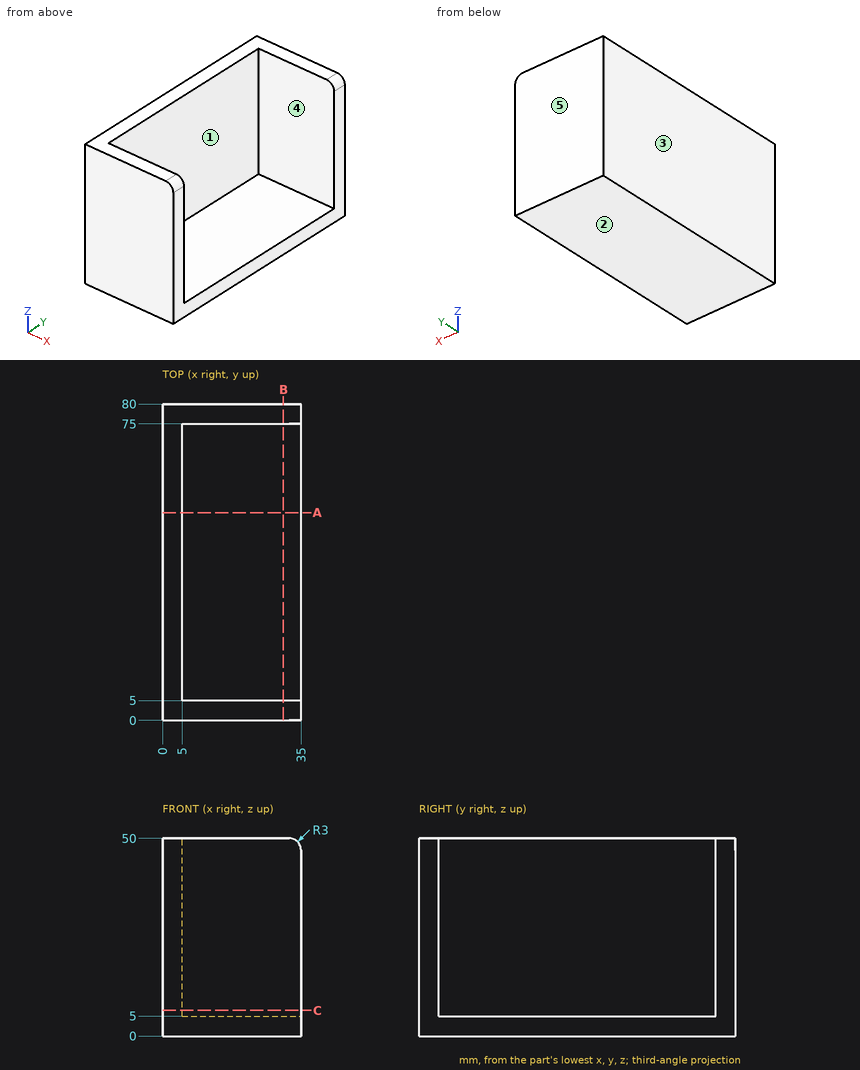
Here's the drawing with two shaded views (mm, measured from the low corner). I have some questions. A direction names the side the tool comes from. Round coordinates to 2 decimals unless told otherwise and drop trailing zeros. Loops run counter-clockwise (first coordinate to the right, second up) from the corner with the lowest first, then second, coordinate; pieces in that order, holes last.
1. Suppose I cut it at B-B, the plane x = 30.5. Please give me the cut outline in (y, z).
Answers:
outline: (0, 0) - (80, 0) - (80, 50) - (75, 50) - (75, 5) - (5, 5) - (5, 50) - (0, 50) - close
2. Suppose I cut it at C-C, the plane z = 6.5. Please give me the cut outline in (x, y), and give its area (3 significant figures).
Answers:
outline: (0, 0) - (35, 0) - (35, 5) - (5, 5) - (5, 75) - (35, 75) - (35, 80) - (0, 80) - close
area: 700 mm2
3. For the marked faces 1 and 2, which set-ups out of +Z, -Z, +X, -X, +Y, -Y let a thin tool reach every point of the face, with its end or its side?
Answers:
face 1: +Z, +X
face 2: -Z, +X, -X, +Y, -Y
4. If I drill on probe 1 along Y at (x, z) = (9, 41); probe 2 along X at (y, z) = (73, 5.5), over which ranges is the centre line in solid material (lowest first)?
Answers:
probe 1: y = 0 to 5, 75 to 80
probe 2: x = 0 to 5
5. Will these pins go through, and if not, where does the flat tip stop? pin 1 (15 mm diameter, centred on x = 16, y = 28.5, fed in from +Z); pin 2 (1.5 mm diameter, centred on y = 61, z = 19.5, fed in from +X).
Answers:
pin 1: stops at z = 5
pin 2: stops at x = 5
6. Suppose I cut it at A-A, the plane y = 52.5. Please give me the cut outline in (x, z).
Answers:
outline: (0, 0) - (35, 0) - (35, 5) - (5, 5) - (5, 50) - (0, 50) - close
7. Thinking about a two-plate mould opening in Y: for the marked faces 3, 4 and 5, which applies, released by +Y, released by -Y, zero draft, split by the parting line, or undercut?
Answers:
face 3: zero draft
face 4: undercut
face 5: released by +Y
